from build123d import *

# Parameters (mm, degrees)
F1_DEPTH = 152.4


# Not quite as in the source:
# - ends of sketch curves that miss each other by under 0.0002 mm in the source are joined


with BuildPart() as f1:
    # F0 (on Front) → F1 (new body)
    with BuildSketch(Plane.XZ):
        with BuildLine():
            ThreePointArc((-21.436008248, 11.1083378523), (-23.575890093, 7.8892124872), (-26.7950133579, 5.7493274827))
            Line((-26.7950133579, 5.7493274827), (-26.7950188, 2.1766784))
            Line((-26.7950188, 2.1766784), (-12.5043438, 2.1766784))
            Line((-12.5043438, 2.1766784), (-12.5043438, -8.5413342))
            Line((-12.5043438, -8.5413342), (0.6985, -14.010132))
            Line((0.6985, -14.010132), (26.7949934, -15.8565596))
            Line((26.7949934, -15.8565596), (26.7949934, -11.9503444))
            ThreePointArc((26.7949934, -11.9503444), (25.7485848099, -9.4240905901), (23.222331, -8.377682))
            ThreePointArc((23.222331, -8.377682), (21.2667719884, -8.9604103578), (19.949146016, -10.5185005939))
            ThreePointArc((19.949146016, -10.5185005939), (19.0509354729, -11.4291461184), (17.7741589903, -11.5058412669))
            ThreePointArc((17.7741589903, -11.5058412669), (7.8088470745, -8.265032818), (3.892042, 1.4544802))
            Line((3.892042, 1.4544802), (0.3963321215, 2.1892390214))
            Line((0.3963321215, 2.1892390214), (0.1486383408, 5.85559709))
            ThreePointArc((0.1486383408, 5.85559709), (-3.4794590188, 13.2572174827), (-11.3164912909, 15.8122126013))
            ThreePointArc((-11.3164912909, 15.8122126013), (-16.0919447869, 13.968734586), (-19.7856463188, 10.4247345468))
            Line((-19.7856463188, 10.4247345468), (-21.436008248, 11.1083378523))
        make_face()
    extrude(amount=F1_DEPTH)


solid = f1.part
Model file for the job. Use its own axes, mm. A direction names the side the tool comes from. Give positions to 0.01 mm unless a question says otherwise; leave off trailing zeros. Write each loop counter-clockwise with the first axis right and the second up, starting at its lowest first coordinate (ties: lowest second). Pieces come first, ordered by that corner, then holes. Notation, with made-up numbers: M -35,-4 L 16,-4 A24 ccw 16,20 Z; hole C 69.5,55.25 d2. An arc over 180 degrees is marked long. One line per item, written item: value. Start each with the question number.
Q1. Saw through at B-B, the plane x = -9. Write the cut outline in (y, z), plus the area to 3 significant figures.
Q2. Probe probe 1 along X at (y, z) = (-108, 0.5); probe 2 along Z at (x, y) = (-3, -68); probe 3 along Z at (x, y) = (22, -142.5). List the from-to ranges inside material, lowest first. Write a range as [from, to].
Q3. 3-axis set-ups, long thin cutter, end or side, ignore diameter. For faces 1 (the flat face through (-20, -75, 2.177)), 2 (the flat face through (-6, -152.4, 0)): which of +Z, -Z, +X, -X, +Y, -Y reach the whole face in a straight line?
Q4. Saw through at C-C, the plane z = 12.5. Write the cut outline in (x, y), plus the area to 3 significant figures.
Q5. Saw through at A-A, the plane y = -139. Write the cut outline in (x, z) (1 decimal).
Q6. Drop flat-ended pins along their axis: pin 1 Ø11.5 at (x, y) = (-23, -73) entering from -Z; pin 2 Ø3 at (x, z) = (7, -1.5) entering from -Y; pin 3 Ø8 at (y, z) = (-57.5, 10) entering from -X; pin 4 Ø1.5 at (y, z) = (-84.5, -4.5) entering from -X. Give the stop position or say it passes through.
Output values:
1. outline: M -152.4,-9.99 L 0,-9.99 L 0,15.75 L -152.4,15.75 Z
1. area: 3,920 mm²
2. probe 1: x = [-12.5, 3.88]
2. probe 2: z = [-12.48, 12.81]
2. probe 3: z = [-15.52, -8.59]
3. face 1: -Z, -X, +Y, -Y
3. face 2: +Z, -Z, +X, -X, -Y
4. outline: M -17.99,-152.4 L -2.69,-152.4 L -2.69,0 L -17.99,0 Z
4. area: 2,330 mm²
5. outline: M -26.8,2.2 L -12.5,2.2 L -12.5,-8.5 L 0.7,-14 L 26.8,-15.9 L 26.8,-12 A3.6 ccw 19.9,-10.5 A1.8 cw 17.8,-11.5 A12.4 cw 3.9,1.5 L 0.4,2.2 L 0.1,5.9 A10.6 ccw -11.3,15.8 A13 ccw -19.8,10.4 L -21.4,11.1 A9.8 cw -26.8,5.7 Z
6. pin 1: stops at z = 2.18
6. pin 2: passes through
6. pin 3: stops at x = -26.23
6. pin 4: stops at x = -12.5
